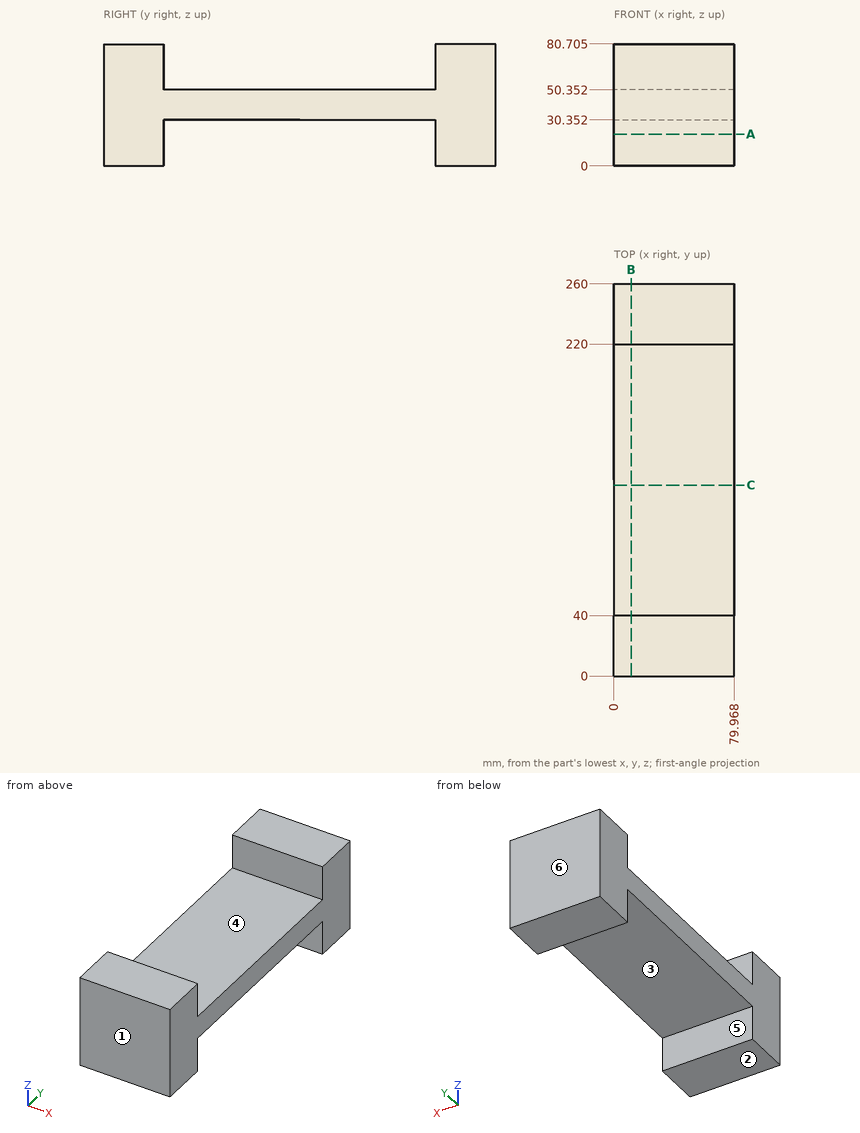
The drawing under review shows one solid part. Ordinate dimensions are in mm from its lowest x, y, z. A direction names the side the tool comes from. Round coordinates to 2 decimals unless told otherwise and drop trailing zeros. Write each loop counter-clockwise with the first axis right and the second up, starting at its lowest first coordinate (ties: lowest second). Pieces come first, ordered by that corner, then holes. Notation, with made-up numbers: M 86,79.5 L 144,79.5 A15 cw 144,92.5 Z; hole C -5,-8.75 d4. An arc over 180 degrees is marked long. One line per item, written item: value. Start each with the question number.
(1) We need section C-C (y = 126.5). Give the boundary of the cut face in (x, z).
(2) The part is to be moulded in two halves that separate along Y. For the marked faces 1, 2 and 3, say which applies: released by +Y, released by -Y, zero draft, split by the parting line, or undercut.
(3) Wall thickness on line 1 (Y direction, x = 67, z = 12); line 2 (Z direction, x = 15.5, y = 154): over which ranges is each line inside the solid? List them lowest first.
(4) We need section B-B (x = 11.5). Give the boundary of the cut face in (y, z) (1 decimal).
(5) We need section A-A (z = 21). Give the boundary of the cut face in (x, y).
(6) Machinability: for the marked faces 4, 5 and 6, which of the approach directions +Z, -Z, +X, -X, +Y, -Y give a long, thin tool a straight path to every point of the face, cutting with its end or side? Answer none if there is none.
(7) Insertion check: pin 1 (12 mm diameter, centred on x = 29.5, y = 93, fed in from -Z); pin 2 (1.5 mm diameter, centred on x = 61, y = 168.5, fed in from +Z). Each pin has a flat end and moves straight along its axis. Give the tip position at first contact, or say it passes through.
Result:
1. outline: M 0,30.35 L 79.97,30.35 L 79.97,50.35 L 0,50.35 Z
2. face 1: released by -Y
2. face 2: zero draft
2. face 3: undercut
3. line 1: 0 to 40, 220 to 260
3. line 2: 30.35 to 50.35
4. outline: M 0,0 L 40,0 L 40,30.4 L 220,30.4 L 220,0 L 260,0 L 260,80.7 L 220,80.7 L 220,50.4 L 40,50.4 L 40,80.7 L 0,80.7 Z
5. outline: M 0,0 L 79.97,0 L 79.97,40 L 0,40 Z; M 0,220 L 79.97,220 L 79.97,260 L 0,260 Z
6. face 4: +Z, +X, -X
6. face 5: -Z, +X, -X
6. face 6: +Z, -Z, +X, -X, +Y
7. pin 1: z = 30.35
7. pin 2: z = 50.35
